Geometry: final body of the model. Coordinates: model frame, mm. A direction names the side the tool comes from. Give positions to 0.01 mm unless a question says otherwise; leave off trailing zeros. Write each loop counter-clockwise with the first axis right and the second up, starting at its lowest first coordinate (ties: lowest second). Pieces come first, ordered by that corner, then holes. Notation, with made-up numbers: M 0,-17 L 42,-17 A15 ccw 42,-6 Z; hole C 83,-22 d10. An arc over 180 degrees is marked long. Use a Markdown table: item, result. Add a question column.
1) Section A-A on x = 0. Return the cut outline in (y, z).
2) Draft query along X for faces 3 (the flat face through (0, 8, -0.25)), 4 (the cylindrical face through (0, 5, 0)). Return one class per face: +X half, -X half, draft (parallel to the pull), parting line (faces both ways), or undercut.
3) Pin query (flat end, axial travel): pin 1 (2.5 mm diameter, centred on x = 9, y = 13.5, fed in from -Z). Return the tip coordinate at first contact, or that it passes through.
4) Section D-D on x = -9. Return the cut outline in (y, z).
5) Section C-C on y = -9.5. Return the cut outline in (x, z), then the cut area to 3 significant figures.
6) Set-up query: faces 1 (the cylindrical face through (6, -5, 0)), 2 (the flat face through (0, 8, 0.25)). Return all of +Z, -Z, +X, -X, +Y, -Y with unobstructed straight access to the full face (end or side cutting, diameter ignored); none if empty.
7) Line query: line 1 (Y direction, x = -21, z = -0.05); line 2 (X direction, y = 0.5, z = 0.2); line 3 (Y direction, x = 9, z = -0.1). Output: solid intervals per line, ascending.
8) Section B-B on z = 0.05. State how many separate pieces and enclosed holes the cut face has, then the cut area to 3 significant figures.
```python
from build123d import *

# Parameters (mm, degrees)
SKETCH1_W           = 55
SKETCH1_H           = 36
SKETCH1_R           = 2
BOSS_EXTRUDE1_DEPTH = 0.25


with BuildPart() as part:
    # Sketch1 → Boss-Extrude1 (new, symmetric)
    with BuildSketch(Plane.XY):
        Rectangle(SKETCH1_W, SKETCH1_H)
        with Locations((-9, 13.5)):
            Circle(SKETCH1_R, mode=Mode.SUBTRACT)
        with Locations((-21, 9.5)):
            Circle(SKETCH1_R, mode=Mode.SUBTRACT)
        with Locations(Location((-9, -13.5, 0), (0, 0, 180))):
            Circle(SKETCH1_R, mode=Mode.SUBTRACT)
        with Locations(Location((-21, -9.5, 0), (0, 0, 180))):
            Circle(SKETCH1_R, mode=Mode.SUBTRACT)
        with Locations((9, -13.5)):
            Circle(SKETCH1_R, mode=Mode.SUBTRACT)
        with Locations((21, -9.5)):
            Circle(SKETCH1_R, mode=Mode.SUBTRACT)
        with Locations(Location((9, 13.5, 0), (0, 0, 180))):
            Circle(SKETCH1_R, mode=Mode.SUBTRACT)
        with Locations(Location((21, 9.5, 0), (0, 0, 180))):
            Circle(SKETCH1_R, mode=Mode.SUBTRACT)
        with BuildLine():
            Line((2.25, 2.75), (2.25, -2.75))
            ThreePointArc((2.25, -2.75), (0, -5), (-2.25, -2.75))
            Line((-2.25, -2.75), (-2.25, 2.75))
            ThreePointArc((-2.25, 2.75), (0, 5), (2.25, 2.75))
        make_face(mode=Mode.SUBTRACT)
        with BuildLine():
            Line((-4.75, 3.75), (-4.75, -3.75))
            ThreePointArc((-4.75, -3.75), (-6, -5), (-7.25, -3.75))
            Line((-7.25, -3.75), (-7.25, 3.75))
            ThreePointArc((-7.25, 3.75), (-6, 5), (-4.75, 3.75))
        make_face(mode=Mode.SUBTRACT)
        with BuildLine():
            Line((4.75, 3.75), (4.75, -3.75))
            ThreePointArc((4.75, -3.75), (6, -5), (7.25, -3.75))
            Line((7.25, -3.75), (7.25, 3.75))
            ThreePointArc((7.25, 3.75), (6, 5), (4.75, 3.75))
        make_face(mode=Mode.SUBTRACT)
    extrude(amount=BOSS_EXTRUDE1_DEPTH, both=True)


solid = part.part
```
Found:
| question | item | result |
|---|---|---|
| 1 | outline | M -18,-0.25 L -5,-0.25 L -5,0.25 L -18,0.25 Z; M 5,-0.25 L 18,-0.25 L 18,0.25 L 5,0.25 Z |
| 2 | face 3 | draft |
| 2 | face 4 | undercut |
| 3 | pin 1 | through |
| 4 | outline | M -18,-0.25 L -15.5,-0.25 L -15.5,0.25 L -18,0.25 Z; M -11.5,-0.25 L 11.5,-0.25 L 11.5,0.25 L -11.5,0.25 Z; M 15.5,-0.25 L 18,-0.25 L 18,0.25 L 15.5,0.25 Z |
| 5 | outline | M -27.5,-0.25 L -23,-0.25 L -23,0.25 L -27.5,0.25 Z; M -19,-0.25 L 19,-0.25 L 19,0.25 L -19,0.25 Z; M 23,-0.25 L 27.5,-0.25 L 27.5,0.25 L 23,0.25 Z |
| 5 | area | 23.5 mm² |
| 6 | face 1 | +Z, -Z |
| 6 | face 2 | +Z, +X, -X, +Y, -Y |
| 7 | line 1 | -18 to -11.5, -7.5 to 7.5, 11.5 to 18 |
| 7 | line 2 | -27.5 to -7.25, -4.75 to -2.25, 2.25 to 4.75, 7.25 to 27.5 |
| 7 | line 3 | -18 to -15.5, -11.5 to 11.5, 15.5 to 18 |
| 8 | separate pieces | 1 |
| 8 | enclosed holes | 11 |
| 8 | area | 1,790 mm² |
